Read the model definition and answer for the solid it produces. Units are mm, in the model's axes. Face numbers are marked on the shaded views. Give positions to 0.01 mm unless a question says otherwise; leave off trailing zeros. Order: outer loops, then holes, each group sorted by start corner. A loop starts at its lowest first (then second) coordinate and runs counter-clockwise, first axis right, second up. Notation, with made-up numbers: (40, 73.5) -> (64, 73.5) arc R19 ccw to (64, 87.5) -> close; hole circle Ø10 at (30.25, 43.25). An arc over 180 degrees is marked (long way). Answer as CSV lines item,"result". Start each with the question number.
1) Flat-ended cylindrical pins translate along their axes: pin 1 Ø6 at (x, z) = (12, -19) entering from +Y; pin 2 Ø2 at (x, z) = (25.5, -4.5) entering from +Y. Find the tip coordinate at first contact, or state that the pin passes through.
2) The mould has two halves that part along X. Classify the marked faces 1, 2, 3 and 4: +X half, -X half, draft (parallel to the pull), parting line (faces both ways), or undercut.
3) Find section C-C (x = 4.5). State how many separate pieces and enclosed holes the cut face has, and give its area (3 significant figures).
4) Straight lines are drawn through the part: L1, parallel to X at y = -7.5, z = -16; L2, parallel to Z at x = 25.5, y = -5.75; L3, parallel to Z at x = 4, y = -8.25. For each, find the intervals that lie inside material, in ascending order. Write a range as from..to.
5) Find section B-B (y = -1). Determine the outline of the cut face in (x, z), and give its area (3 significant figures).
```python
from build123d import *

# Parameters (mm, degrees)
F0_W     = 30
F0_H     = 30
F0_R     = 10
F0_R_2   = 3
F1_DEPTH = 12
F2_DEPTH = 3
F3_R     = 0.2
F4_R     = 12
F4_R_2   = 11
F5_DEPTH = 0.6
F6_R     = 0.49999
F4_R_3   = 1.25
F7_DEPTH = 25
F8_SIZE  = 0.25


# Not quite as in the source:
# - a fillet or chamfer is up to 0.001 mm smaller than in the source, because OpenCascade refuses the exact size


with BuildPart() as f1:
    # F0 (on Front) → F1 (new body)
    with BuildSketch(Plane.XZ):
        with Locations((15, -15)):
            Rectangle(F0_W, F0_H)
        with Locations((15, -15)):
            Circle(F0_R, mode=Mode.SUBTRACT)
        with Locations((15, -15)):
            Circle(F0_R)
        with Locations((15, -16.066)):
            Circle(F0_R_2, mode=Mode.SUBTRACT)
    extrude(amount=F1_DEPTH)

    # F0 (on Front) → F2 (cut)
    with BuildSketch(Plane.XZ):
        with Locations((15, -15)):
            Circle(F0_R)
        with Locations((15, -16.066)):
            Circle(F0_R_2, mode=Mode.SUBTRACT)
    extrude(amount=F2_DEPTH, mode=Mode.SUBTRACT)

    # F3
    f3_edges = [f1.edges().sort_by_distance(p)[0] for p in [
        (5, -3, -15),
    ]]
    fillet(f3_edges, radius=F3_R)

    # F4 (on face) → F5 (cut)
    with BuildSketch(Plane(origin=(0, 0, 0), x_dir=(-1, 0, 0), z_dir=(0, 1, 0))):
        with Locations((-15, -15)):
            Circle(F4_R)
        with Locations((-15, -15)):
            Circle(F4_R_2, mode=Mode.SUBTRACT)
    extrude(amount=-F5_DEPTH, mode=Mode.SUBTRACT)

    # F6 (radius 0.5 in the source; OpenCascade refuses exactly that, so slightly less here)
    f6_edges = [f1.edges().sort_by_distance(p)[0] for p in [
        (26, -0.6, -15),
        (27, -0.6, -15),
    ]]
    fillet(f6_edges, radius=F6_R)

    # F4 (on face) → F7 (cut)
    with BuildSketch(Plane(origin=(0, 0, 0), x_dir=(-1, 0, 0), z_dir=(0, 1, 0))):
        with Locations((-4.5, -4.5)):
            Circle(F4_R_3)
        with Locations((-25.5, -4.5)):
            Circle(F4_R_3)
        with Locations((-25.5, -25.5)):
            Circle(F4_R_3)
        with Locations((-4.5, -25.5)):
            Circle(F4_R_3)
    extrude(amount=-F7_DEPTH, mode=Mode.SUBTRACT)

    # F8
    f8_edges = [f1.edges().sort_by_distance(p)[0] for p in [
        (15, -12, 0),
        (30, -12, -15),
        (0, -12, -15),
        (15, -12, -30),
        (5.75, -12, -25.5),
        (26.75, -12, -25.5),
        (12, -12, -16.066),
        (5.75, -12, -4.5),
        (26.75, -12, -4.5),
        (30, -6, 0),
        (0, -6, 0),
        (30, -6, -30),
        (0, -6, -30),
        (5.75, 0, -4.5),
        (3.25, -6, -4.5),
        (26.75, 0, -25.5),
        (5.75, 0, -25.5),
        (3.25, -6, -25.5),
        (26.75, 0, -4.5),
    ]]
    chamfer(f8_edges, length=F8_SIZE)


solid = f1.part
```
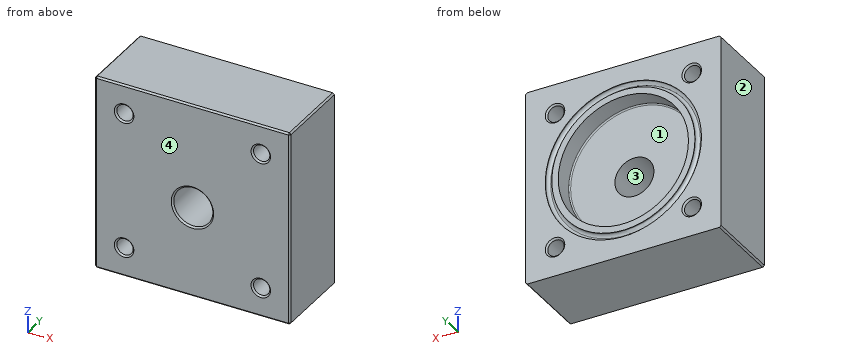
Findings below:
1,pin 1,"y = -3"
1,pin 2,"through"
2,face 1,"undercut"
2,face 2,"-X half"
2,face 3,"undercut"
2,face 4,"draft"
3,separate pieces,"3"
3,enclosed holes,"0"
3,area,"297 mm²"
4,L1,"0..12, 18..30"
4,L2,"-30..-26.75, -24.25..-5.75, -3.25..0"
4,L3,"-30..-26.65, -24.35..-5.65, -3.35..0"
5,outline,"(0, -29.75) -> (0.25, -30) -> (29.75, -30) -> (30, -29.75) -> (30, -0.25) -> (29.75, 0) -> (0.25, 0) -> (0, -0.25) -> close; hole circle Ø2.5 at (4.5, -25.5); hole circle Ø2.5 at (4.5, -4.5); hole circle Ø20 at (15, -15); hole circle Ø2.5 at (25.5, -25.5); hole circle Ø2.5 at (25.5, -4.5)"
5,area,"566 mm²"
